Could you check a few things on this model? Use its own coordinates, in mm. A direction names the side the tool comes from. Round coordinates to 2 decimals unless told otherwise and drop trailing zeros. Loops run counter-clockwise (first coordinate to the right, second up) from the corner with the lowest first, then second, coordinate; pieces in that order, holes last. Notation, with made-up numbers: (41.25, 16.5) - (62.25, 16.5) arc R25 cw to (62.25, 45.5) - close; hole circle Ø4 at (31.25, 29.25). An arc over 180 degrees is marked (long way). Answer as CSV lines item,"result". Start each with the question number.
1) We'd pull the mould along Z, two halves only. Please class faces 4 (the face through (0, 0, 8.7)), 5 (the face through (0, 0, 1.2)), 6 (the face through (0, 0, 0)), 7 (the face through (7.62, -3.16, 0.59)): pulls with the +Z half, pulls with the -Z half, needs draft (parallel to the pull), parting line crosses it, or undercut.
2) Please list where these lines run through material, in increasing order: line 1 along Z through (x, y) = (0.75, 0.25); line 2 along Z through (x, y) = (-5.5, -4); line 3 along Y through (x, z) = (0.75, 7).
3) Suppose I cut it at D-D, the plane x = 7.25. Write out the boundary of the cut face in (y, z), then the cut area to 3 significant figures.
4) I'm going to push flat-ended pins straight in: pin 1 Ø4 at (x, z) = (-0.5, 6) entering from +Y; pin 2 Ø1 at (x, z) = (5, 5.5) entering from -Y; pin 3 Ø3 at (x, y) = (2, -2.5) entering from -Z. Where does each tip first touch, or does it pass through?
5) Which directions (+Z, -Z, +X, -X, +Y, -Y) give clear straight access to the entire face, cutting with the end or side of a thin tool? Please do faces 1 (the face through (-4, 6, 1.2)), 2 (the face through (0, 0.75, 1)), 3 (the face through (0, 0, 9.5)).
6) Suppose I cut it at C-C, the plane z = 7.5. Write out the boundary of the cut face in (x, y), then the cut area to 3 significant figures.
7) Suppose I cut it at A-A, the plane x = 0. Write out the boundary of the cut face in (y, z), then the cut area to 3 significant figures.
8) Suppose I cut it at B-B, the plane z = 2.5. Write out the boundary of the cut face in (x, y).
```python
from build123d import *

# Parameters (mm, degrees)
F1_DEPTH = 9.5
F2_T     = -0.8
F0_R     = 8.25
F3_DEPTH = 1.2
F4_SIZE2 = 2.2860104606
F4_SIZE  = 0.2
F5_SIZE  = 0.5


with BuildPart() as f1:
    # F0 (on Top) → F1 (new body)
    with BuildSketch(Plane.XY):
        with BuildLine():
            ThreePointArc((6.0537178659, -0.75), (6.0884184721, -0.3757133335), (6.1, 0))
            ThreePointArc((6.1, 0), (6.0884184721, 0.3757133335), (6.0537178659, 0.75))
            Line((6.0537178659, 0.75), (-6.0537178659, 0.75))
            ThreePointArc((-6.0537178659, 0.75), (-6.1, 0), (-6.0537178659, -0.75))
            Line((-6.0537178659, -0.75), (6.0537178659, -0.75))
        make_face()
        with BuildLine():
            Line((-6.0537178659, 0.75), (6.0537178659, 0.75))
            ThreePointArc((6.0537178659, 0.75), (0, 6.1), (-6.0537178659, 0.75))
        make_face()
        with BuildLine():
            ThreePointArc((-6.0537178659, -0.75), (0, -6.1), (6.0537178659, -0.75))
            Line((6.0537178659, -0.75), (-6.0537178659, -0.75))
        make_face()
    extrude(amount=F1_DEPTH)

    # F2
    f2_openings = [f1.faces().sort_by_distance(p)[0] for p in [
        (0, 0, 0),
    ]]
    offset(amount=F2_T, openings=f2_openings)

    # F0 (on Top) → F3 (join)
    with BuildSketch(Plane.XY):
        Circle(F0_R)
        with BuildLine():
            ThreePointArc((-6.0537178659, 0.75), (0, 6.1), (6.0537178659, 0.75))
            Line((6.0537178659, 0.75), (7.5, 0.75))
            Line((7.5, 0.75), (7.5, -0.75))
            Line((7.5, -0.75), (6.0537178659, -0.75))
            ThreePointArc((6.0537178659, -0.75), (0, -6.1), (-6.0537178659, -0.75))
            Line((-6.0537178659, -0.75), (-7.5, -0.75))
            Line((-7.5, -0.75), (-7.5, 0.75))
            Line((-7.5, 0.75), (-6.0537178659, 0.75))
        make_face(mode=Mode.SUBTRACT)
        with BuildLine():
            ThreePointArc((6.0537178659, -0.75), (6.0884184721, -0.3757133335), (6.1, 0))
            ThreePointArc((6.1, 0), (6.0884184721, 0.3757133335), (6.0537178659, 0.75))
            Line((6.0537178659, 0.75), (-6.0537178659, 0.75))
            ThreePointArc((-6.0537178659, 0.75), (-6.1, 0), (-6.0537178659, -0.75))
            Line((-6.0537178659, -0.75), (6.0537178659, -0.75))
        make_face()
        with BuildLine():
            ThreePointArc((6.0537178659, 0.75), (6.0884184721, 0.3757133335), (6.1, 0))
            ThreePointArc((6.1, 0), (6.0884184721, -0.3757133335), (6.0537178659, -0.75))
            Line((6.0537178659, -0.75), (7.5, -0.75))
            Line((7.5, -0.75), (7.5, 0.75))
            Line((7.5, 0.75), (6.0537178659, 0.75))
        make_face()
        with BuildLine():
            ThreePointArc((-6.0537178659, -0.75), (-6.1, 0), (-6.0537178659, 0.75))
            Line((-6.0537178659, 0.75), (-7.5, 0.75))
            Line((-7.5, 0.75), (-7.5, -0.75))
            Line((-7.5, -0.75), (-6.0537178659, -0.75))
        make_face()
    extrude(amount=F3_DEPTH)

    # F4
    f4_edges = [f1.edges().sort_by_distance(p)[0] for p in [
        (6.053718, 0.75, 9.5),
    ]]
    f4_side = f1.faces().sort_by_distance((0, 0, 9.5))[0]
    chamfer(f4_edges, length=F4_SIZE, length2=F4_SIZE2, reference=f4_side)

    # F5
    f5_edges = [f1.edges().sort_by_distance(p)[0] for p in [
        (6.053718, 0.75, 1.2),
    ]]
    chamfer(f5_edges, length=F5_SIZE)


solid = f1.part
```
Filled sheet:
1,face 4,"undercut"
1,face 5,"undercut"
1,face 6,"pulls with the -Z half"
1,face 7,"needs draft"
2,line 1,"0 to 1.2, 8.7 to 9.5"
2,line 2,"0 to 1.2"
2,line 3,"-6.05 to -5.25, 5.25 to 6.05"
3,outline,"(-3.94, 0) - (3.94, 0) - (3.94, 1.2) - (-3.94, 1.2) - close"
3,area,"9.45 mm²"
4,pin 1,"y = 6.1"
4,pin 2,"y = -4.12"
4,pin 3,"z = 8.7"
5,face 1,"+Z"
5,face 2,"-Z"
5,face 3,"+Z, +X, -X, +Y, -Y"
6,outline,"circle Ø12.15 at (0, 0); hole circle Ø10.6 at (0, 0)"
6,area,"27.7 mm²"
7,outline,"(-8.25, 0) - (-5.3, 0) - (-5.3, 8.7) - (5.3, 8.7) - (5.3, 0) - (8.25, 0) - (8.25, 1.2) - (6.6, 1.2) - (6.1, 1.7) - (6.1, 7.21) - (5.9, 9.5) - (-5.9, 9.5) - (-6.1, 7.21) - (-6.1, 1.7) - (-6.6, 1.2) - (-8.25, 1.2) - close; (-0.75, 0) - (0.75, 0) - (0.75, 1.2) - (-0.75, 1.2) - close"
7,area,"30.4 mm²"
8,outline,"circle Ø12.2 at (0, 0); hole circle Ø10.6 at (0, 0)"
